Drawing for the job (mm, zero at the part's lowest x, y, z). A direction names the side the tool comes from. Coordinates: 2 decimals unless noted, no trailing zeros. Write each loop counter-clockwise with the first axis right and the second up, starting at its lowest first coordinate (ties: lowest second). Pieces come first, ordered by that corner, then holes. Notation, with made-up numbers: (-5, 77) -> (29, 77) arc R10 ccw to (29, 89) -> close; hole circle Ø4 at (4, 52). An arc over 180 degrees is marked (long way). Write each question's results on one line, items separated by ' | '. Start each with the question number.
Q1. Saw through at B-B on y = 20.75. Give the cut face in (x, z).
Q2. Drill centre lines: line 1 (Y direction, x = 9.25, z = 6.5); line 2 (Y direction, x = 6.5, z = 4.25); line 3 (X direction, y = 6.25, z = 5.5). Where is each one in solid material? Low to high.
Q3. Saw through at D-D on z = 1.5. Give the cut face in (x, y) (3 decimals).
Q4. Saw through at C-C on x = 9.25. Give the cut face in (y, z), and give its area (3 significant figures).
Q5. Two-plate mould, pull along X, no slides. Class the marked faces 1, 2, 3 and 4: released by +X, released by -X, zero draft, split by the parting line, or undercut.
Q6. Saw through at A-A on z = 5.5. Give the cut face in (x, y) (3 decimals).
Q7. Drop flat-ended pins along their axis: pin 1 Ø2 at (y, z) = (6.5, 9.5) entering from +X; pin 2 Ø2 at (y, z) = (17.5, 8) entering from +X; pin 3 Ø3 at (y, z) = (16.5, 4.5) entering from -X. Give the stop position or say it passes through.
Q8. Tool access for the marked faces 5 and 6: list every direction of +Z, -Z, +X, -X, +Y, -Y with a clear straight run to the whole face (end or side of a thin tool).
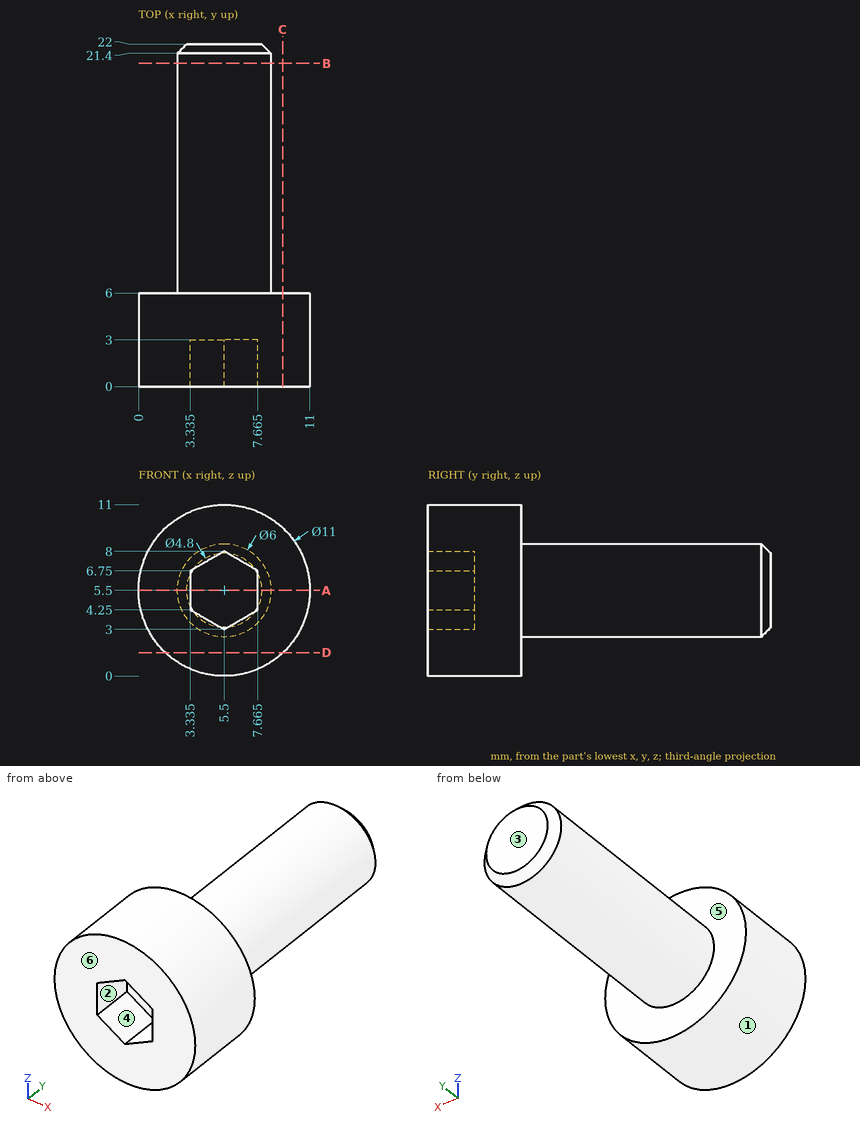
Returned:
1) outline: circle Ø6 at (5.5, 5.5)
2) line 1: y = 0 to 6 | line 2: y = 3 to 22 | line 3: x = 2.5 to 8.5
3) outline: (1.725, 0) -> (9.275, 0) -> (9.275, 6) -> (1.725, 6) -> close
4) outline: (0, 1.48) -> (6, 1.48) -> (6, 9.52) -> (0, 9.52) -> close | area: 48.3 mm2
5) face 1: split by the parting line | face 2: undercut | face 3: zero draft | face 4: undercut
6) outline: (0, 0) -> (3.335, 0) -> (3.335, 3) -> (7.665, 3) -> (7.665, 0) -> (11, 0) -> (11, 6) -> (8.5, 6) -> (8.5, 21.4) -> (7.9, 22) -> (3.1, 22) -> (2.5, 21.4) -> (2.5, 6) -> (0, 6) -> close
7) pin 1: stops at x = 10.02 | pin 2: stops at x = 8.1 | pin 3: stops at x = 2.5
8) face 5: +Y | face 6: +Z, -Z, +X, -X, -Y
